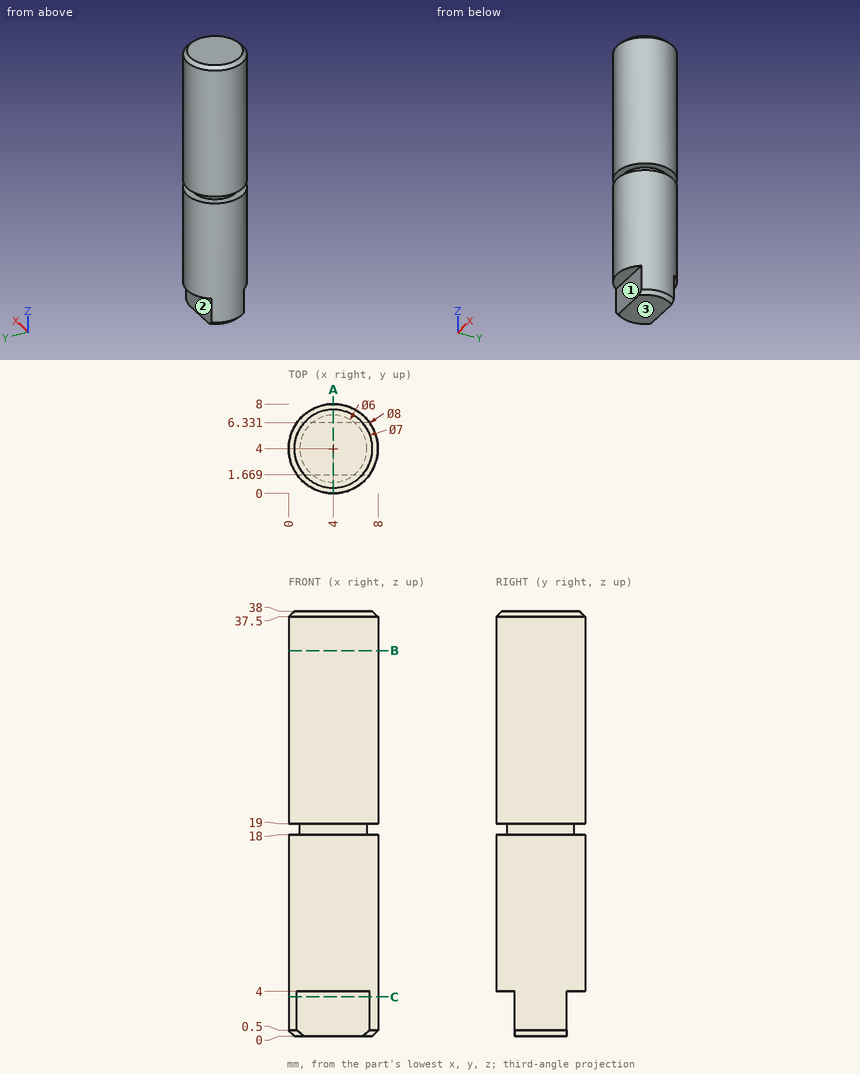
Check sheet for the drawn part. Datum: minimum x, y, z corner. Units: mm. A direction names the side the tool comes from. Give positions to 0.01 mm unless a question says otherwise; leave off trailing zeros. Write each loop counter-clockwise with the first axis right and the second up, starting at its lowest first coordinate (ties: lowest second). Pieces come first, ordered by that corner, then holes. Notation, with made-up numbers: (61.5, 88) - (112.5, 88) arc R21 ccw to (112.5, 126) - close; hole circle Ø9 at (22.5, 54.5). An arc over 180 degrees is marked (long way). Put each result on its own line as item: value.
1. Go/stop test with flat-tipped pins: pin 1 (3 mm diameter, centred on x = 1, z = 30.5, fed in from -Y); pin 2 (3 mm diameter, centred on x = 3.5, z = 1.5, fed in from -Y); pin 3 (3 mm diameter, centred on x = 4, z = 1.5, fed in from +Y). Record where each tip stops, or that it passes through.
Ans:
pin 1: stops at y = 0.29
pin 2: stops at y = 1.67
pin 3: stops at y = 6.33
2. Sectioned sample at B-B, the plane z = 34.5. Enter the section's corners in (x, y).
Ans:
outline: circle Ø8 at (4, 4)
3. Sectioned sample at A-A, the plane x = 4. Enter the section's corners in (y, z), plus the area to 3 significant figures.
Ans:
outline: (0, 4) - (1.67, 4) - (1.67, 0) - (6.33, 0) - (6.33, 4) - (8, 4) - (8, 18) - (7, 18) - (7, 19) - (8, 19) - (8, 37.5) - (7.5, 38) - (0.5, 38) - (0, 37.5) - (0, 19) - (1, 19) - (1, 18) - (0, 18) - close
area: 288 mm²
4. Thickness scan on line 1 (Z direction, x = 7, y = 3.5); line 2 (Z direction, x = 3.75, y = 6.5); line 3 (Z direction, x = 2.75, y = 0.75). Record the ranges inside material, lowest first.
Ans:
line 1: z = 0 to 18, 19 to 38
line 2: z = 4 to 38
line 3: z = 4 to 18, 19 to 38
5. Sectioned sample at C-C, the plane z = 3.5. Enter the section's corners in (x, y).
Ans:
outline: (0.75, 1.67) - (7.25, 1.67) arc R4 ccw to (7.25, 6.33) - (0.75, 6.33) arc R4 ccw to start
6. Set-up check for the marked faces 1, 2 and 3: record each of +Z, -Z, +X, -X, +Y, -Y from which the full face is reachable in a straight line by a thin tool's end or side.
Ans:
face 1: -Z, +X, -X, -Y
face 2: -Z, +X, -X, +Y
face 3: -Z, +X, -X, +Y, -Y
